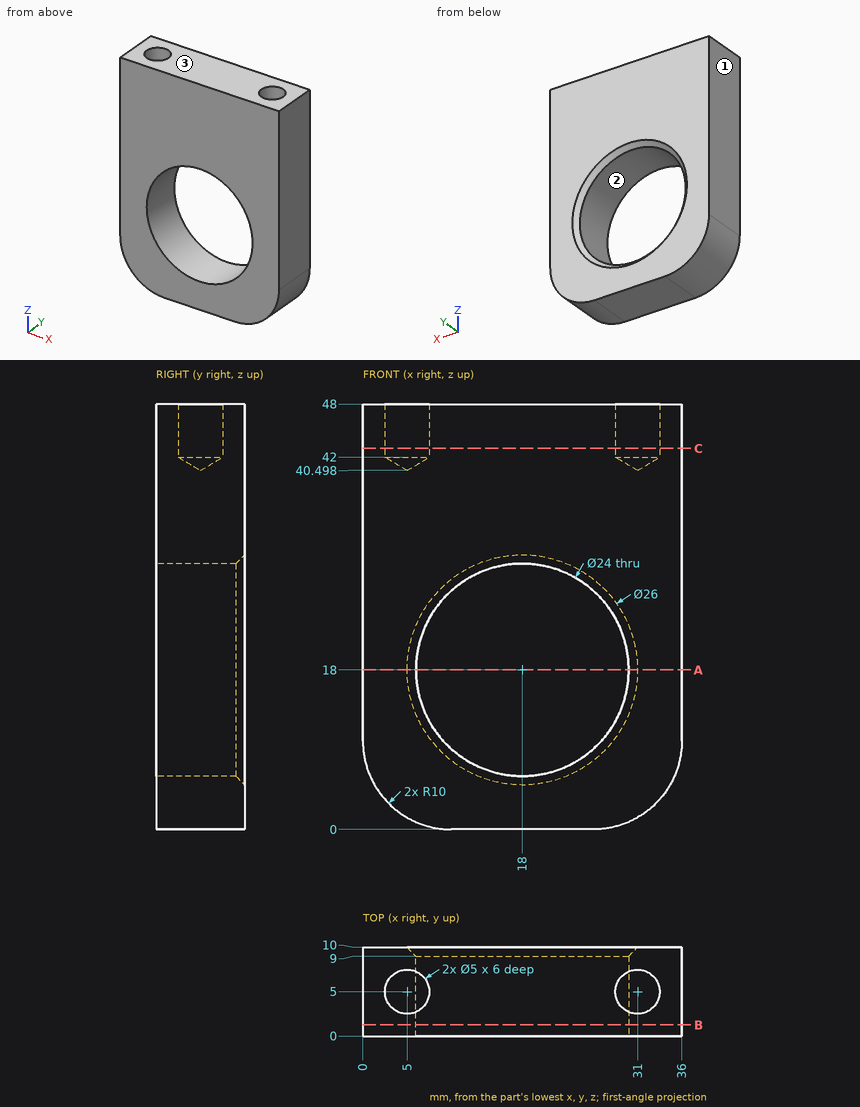
The drawing under review shows one solid part. Ordinate dimensions are in mm from its lowest x, y, z. Coordinates: 2 decimals unless noted, no trailing zeros. Order: outer loops, then holes, each group sorted by start corner. A loop starts at its lowest first (then second) coordinate and runs counter-clockwise, first axis right, second up. Notation, with made-up numbers: (30, 31.25) -> (69, 31.25) arc R5 cw to (69, 35.25) -> close; hole circle Ø10 at (-39.5, 52). An arc over 180 degrees is marked (long way). One line per item, written item: value.
1) To check wall thickness, follow probe 1 along X at (y, z) = (5, 45.3); probe 2 along X at (y, z) = (6.75, 18); probe 3 along X at (y, z) = (3.5, 45.5). State the ranges of each line that lie inside material, in increasing order. Write a range as [from, to].
Output values:
probe 1: x = [0, 2.5], [7.5, 28.5], [33.5, 36]
probe 2: x = [0, 6], [30, 36]
probe 3: x = [0, 3], [7, 29], [33, 36]
2) Clearance check with flat-ended pins moving along their axes: P1, Ø3, axis at x = 13, z = 10.5, coming from the -Y side; P2, Ø3, axis at x = 31, y = 5, coming from the +Z side; P3, Ø4.5, axis at x = 5, y = 5, coming from the -Z side. State where each tip first meets the part, or that it passes through.
Output values:
P1: passes through
P2: stops at z = 41.4
P3: stops at z = 0.39
3) We need section A-A, the plane z = 18. Give the boundary of the cut face in (x, y), then the cut area to 3 significant figures.
Output values:
outline: (0, 0) -> (6, 0) -> (6, 9) -> (5, 10) -> (0, 10) -> close; (30, 0) -> (36, 0) -> (36, 10) -> (31, 10) -> (30, 9) -> close
area: 119 mm2
4) Draft analysis for pull direction Z (two halves, no side actions). For the marked faces 1, 2 and 3, state which applies: +Z half, -Z half, draft (parallel to the pull), parting line (faces both ways), or undercut.
Output values:
face 1: draft
face 2: undercut
face 3: +Z half
5) We need section B-B, the plane y = 1.25. Give the boundary of the cut face in (x, z), then the cut area to 3 significant figures.
Output values:
outline: (0, 10) arc R10 ccw to (10, 0) -> (26, 0) arc R10 ccw to (36, 10) -> (36, 48) -> (0, 48) -> close; hole circle Ø24 at (18, 18)
area: 1,230 mm2
6) We need section C-C, the plane z = 43. Give the boundary of the cut face in (x, y).
Output values:
outline: (0, 0) -> (36, 0) -> (36, 10) -> (0, 10) -> close; hole circle Ø5 at (5, 5); hole circle Ø5 at (31, 5)
